Autodesk Inventor part; units mm, degrees
ref_plane "YZ Plane" through (0, 0, 0) normal (1, 0, 0) x (0, 1, 0)
ref_plane "XZ Plane" through (0, 0, 0) normal (0, 1, 0) x (-1, 0, 0)
ref_plane "XY Plane" through (0, 0, 0) normal (0, 0, 1) x (1, 0, 0)
sketch "Sketch1" plane through (0, 0, 0) normal (0, 0, 1) x (1, 0, 0)
  line L0 (-100, -75) -> (100, -75)
  line L1 (100, -75) -> (100, 75)
  line L2 (100, 75) -> (-100, 75)
  line L3 (-100, 75) -> (-100, -75)
  line L4 (-70, -60) -> (55, -60)
  line L5 (55, 60) -> (-70, 60)
  line L6 (-70, 60) -> (-70, 15)
  line L7 (-70, -15) -> (-70, -60)
  line L8 (151.2343, 15) -> (1.2343, 15)
  line L9 (1.2343, -15) -> (151.2343, -15)
  line L10 (85, -30) -> (85, -15)
  line L11 (85, 15) -> (85, 30)
  line L12 (-100, 75) -> (72.5, 75)
  line L13 (72.5, -75) -> (-100, -75)
  line L14 (-100, -75) -> (-100, 75)
  line L15 (100, -15) -> (85, -15)
  line L16 (100, 15) -> (85, 15)
  line L17 (-100, 0) -> (100, 0) construction
  line L18 (70, 45) -> (70, -45)
  line L19 (70, -45) -> (-70, -45)
  line L20 (-70, -45) -> (-70, 45)
  line L21 (-70, 45) -> (70, 45)
  line L22 (-70, 15) -> (-70, -15)
  line L23 (85, -30) -> (70, -45)
  line L24 (70, -45) -> (55, -45)
  line L25 (55, -45) -> (55, -60)
  line L26 (85, 30) -> (70, 45)
  line L27 (70, 45) -> (55, 45)
  line L28 (55, 45) -> (55, 60)
  line L29 (100, -102.5) -> (110, -102.5)
  line L30 (115, -97.5) -> (115, -67.5)
  line L31 (110, -102.5) -> (115, -97.5)
  line L32 (100, -15) -> (115, -15)
  line L33 (115, -67.5) -> (115, -15)
  line L34 (72.5, -75) -> (72.5, -92.5)
  line L35 (82.5, -102.5) -> (100, -102.5)
  line L36 (72.5, -92.5) -> (82.5, -102.5)
  line L37 (100, 102.5) -> (110, 102.5)
  line L38 (115, 97.5) -> (115, 67.5)
  line L39 (110, 102.5) -> (115, 97.5)
  line L40 (100, 15) -> (115, 15)
  line L41 (115, 67.5) -> (115, 15)
  line L42 (72.5, 75) -> (72.5, 92.5)
  line L43 (82.5, 102.5) -> (100, 102.5)
  line L44 (72.5, 92.5) -> (82.5, 102.5)
  line L45 (270, -60) -> (395, -60)
  line L46 (395, 60) -> (270, 60)
  line L47 (270, 60) -> (270, 15)
  line L48 (270, -15) -> (270, -60)
  line L49 (425, -30) -> (425, -15)
  line L50 (425, 15) -> (425, 30)
  line L51 (240, 75) -> (412.5, 75)
  line L52 (412.5, -75) -> (240, -75)
  line L53 (240, -75) -> (240, 75)
  line L54 (440, -15) -> (425, -15)
  line L55 (440, 15) -> (425, 15)
  line L56 (240, 0) -> (440, 0) construction
  line L57 (270, 15) -> (270, -15)
  line L58 (425, -30) -> (410, -45)
  line L59 (410, -45) -> (395, -45)
  line L60 (395, -45) -> (395, -60)
  line L61 (395, 45) -> (395, 60)
  line L62 (410, 45) -> (395, 45)
  line L63 (425, 30) -> (410, 45)
  line L64 (440, -102.5) -> (450, -102.5)
  line L65 (455, -97.5) -> (455, -67.5)
  line L66 (450, -102.5) -> (455, -97.5)
  line L67 (440, -15) -> (455, -15)
  line L68 (455, -67.5) -> (455, -15)
  line L69 (412.5, -75) -> (412.5, -92.5)
  line L70 (422.5, -102.5) -> (440, -102.5)
  line L71 (412.5, -92.5) -> (422.5, -102.5)
  line L72 (412.5, 75) -> (412.5, 92.5)
  line L73 (412.5, 92.5) -> (422.5, 102.5)
  line L74 (422.5, 102.5) -> (440, 102.5)
  line L75 (440, 102.5) -> (450, 102.5)
  line L76 (450, 102.5) -> (455, 97.5)
  line L77 (455, 97.5) -> (455, 67.5)
  line L78 (455, 67.5) -> (455, 15)
  line L79 (440, 15) -> (455, 15)
  point P0 (0, 0)
  point P1 (85, -60)
  point P2 (85, 60)
  point P3 (100, 15)
  point P4 (100, -15)
  point P5 (-70, 15)
  point P6 (85, -22.5)
  point P7 (70, 15)
  point P8 (70, -15)
  point P9 (115, -102.5)
  point P10 (100, -55)
  point P11 (107.5, 75)
  point P12 (107.5, 95)
  point P13 (107.5, -75)
  point P14 (107.5, -95)
  point P15 (72.5, -102.5)
  point P16 (425, -60)
  point P17 (425, 60)
  point P18 (425, -22.5)
  point P19 (455, -102.5)
  point P20 (447.5, 75)
  point P21 (447.5, 95)
  point P22 (447.5, -95)
  point P23 (447.5, -75)
  point P24 (412.5, -102.5)
  dimension "d3" = 15
  dimension "d4" = 15
  dimension "d5" = 30
  dimension "d13" = 30
  dimension "d17" = 5
  dimension "d18" = 5
  dimension "d74" = 20
  dimension "d76" = 150
  dimension "d78" = 27.5
  dimension "d79" = 10
  dimension "d80" = 10
  dimension "d81" = 215
  dimension "d94" = 15
  dimension "d95" = 30
  dimension "d96" = 5
  dimension "d97" = 5
  dimension "d98" = 20
  dimension "d99" = 150
  dimension "d100" = 27.5
  dimension "d101" = 10
  dimension "d102" = 10
  dimension "d103" = 215
extrude "Extrusion1" add sketch "Sketch1" along normal blind 7 contours L3 L2 L1 L8 L11 L26 L21 L28 L5 L6 L20 L7 L4 L25 L19 L23 L10 L9 L0 | L0 L1 L9 L33 L30 L31 L29 L35 L36 L34 | L42 L44 L43 L37 L39 L38 L41 L8 L1 L2
sketch "Sketch2" plane through (0, 0, 7) normal (0, 0, 1) x (1, 0, 0)
  line L0 (-70, -60) -> (-70, 60) construction
  line L1 (-70, 0) -> (130.7679, 0) construction
  line L2 (115, -97.5) -> (115, -15) construction
  line L3 (-100, -102.5) -> (110, -102.5) construction
  line L4 (115, -15) -> (85, -15) construction
  point P0 (0, 0)
  point P1 (107.5, -75)
  point P2 (107.5, -95)
  point P3 (107.5, 75)
  point P4 (107.5, 95)
  point P5 (115, -20)
  point P6 (-100, -75)
  point P7 (110, -15)
  point P8 (115, -20)
  point P9 (100, -15)
  dimension "d21" = 7.5
  dimension "d24" = 7.5
  dimension "d32" = 20
  dimension "d73" = 150
hole "Hole1" at (107.5, -75, 7) at (107.5, -95, 7) at (107.5, 75, 7) at (107.5, 95, 7) direction (0, 0, -1) diameter 4 end through all
properties part number "Marco" material "MDF Medium Density Fiberboard"
Work out the finished part from the listing and answer in its coordinate system (mm). A direction names the side the tool comes from. Give positions to 0.01 mm unless a question says otherwise; leave off trailing zeros. Write each loop counter-clockwise with the first axis right and the second up, starting at its lowest first coordinate (ties: lowest second). Pieces come first, ordered by that corner, then holes.
(1) The part is cut by section B-B on x = 45. Write down the section's boundary in (y, z).
Final values:
outline: (-75, 0) - (-60, 0) - (-60, 7) - (-75, 7) - close; (60, 0) - (75, 0) - (75, 7) - (60, 7) - close
(2) Which of the six approach directions +Z, -Z, +X, -X, +Y, -Y give full straight-line access (tool end or side, diameter ignored) to faces 4 (the flat face through (96, -102.5, 3)), 5 (the flat face through (-13, 75, 3)), 6 (the flat face through (63, -45, 3)), 7 (the flat face through (-15, -75, 3))?
Final values:
face 4: +Z, -Z, +X, -X, -Y
face 5: +Z, -Z, -X, +Y
face 6: +Z, -Z
face 7: +Z, -Z, -X, -Y
(3) Straight lines are drawn through the part: line 1 (Y direction, x = 107.5, z = 4.5); line 2 (Y direction, x = -45.5, z = 3.25); line 3 (X direction, y = -54.5, z = 6). For each, find the intervals that lie inside material, in ascending order.
Final values:
line 1: y = -102.5 to -97, -93 to -77, -73 to -15, 15 to 73, 77 to 93, 97 to 102.5
line 2: y = -75 to -60, 60 to 75
line 3: x = -100 to -70, 55 to 115
(4) The part is cut by section C-C on y = 1.5. Write down the section's boundary in (x, z), plus the area to 3 significant figures.
Final values:
outline: (-100, 0) - (-70, 0) - (-70, 7) - (-100, 7) - close
area: 210 mm2
(5) Flat-ended cylindrical pins translate along their axes: pin 1 Ø2.5 at (x, y) = (107.5, -95) entering from +Z; pin 2 Ø2 at (x, z) = (-50.5, 2.5) entering from -Y; pin 3 Ø3.5 at (x, z) = (-38.5, 5) entering from +Y. Find the tip coordinate at first contact, or state that the pin passes through.
Final values:
pin 1: passes through
pin 2: stops at y = -75
pin 3: stops at y = 75
(6) The mould has two halves that part along Y. Classify faces 1 (the flat face through (78, -37, 3)), 2 (the flat face through (-100, 1, 3)), 3 (the flat face through (77, 97, 3)): pulls with the +Y half, pulls with the -Y half, needs draft (parallel to the pull), parting line crosses it, or undercut.
Final values:
face 1: undercut
face 2: needs draft
face 3: pulls with the +Y half
(7) The part is cut by section A-A on z = 3.75. Count the separate pieces of the cut face and the enclosed holes in it, plus the area to 3 significant figures.
Final values:
separate pieces: 1
enclosed holes: 4
area: 16,000 mm2
